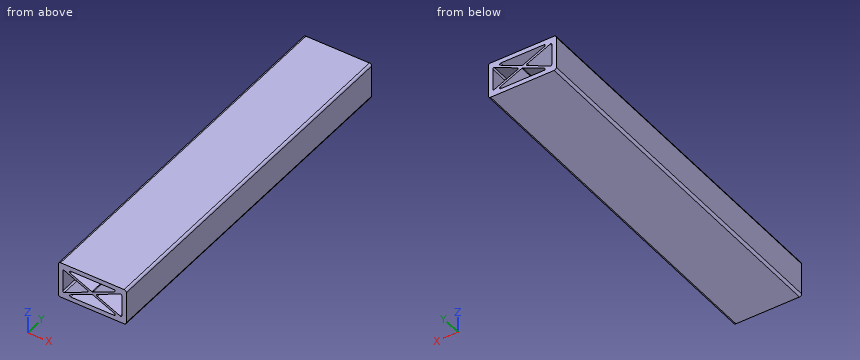
```python
from build123d import *

# Parameters (mm, degrees)
F0_W     = 150
F0_H     = 80
F1_DEPTH = 800
F3_DEPTH = 800.001
F4_R     = 2.5
F5_R     = 5


with BuildPart() as f1:
    # F0 (on Front) → F1 (new body)
    with BuildSketch(Plane.XZ):
        Rectangle(F0_W, F0_H)
    extrude(amount=F1_DEPTH)

    # F2 (on face) → F3 (cut, through all)
    with BuildSketch(Plane.XZ.offset(800)):
        Polygon((59.034241, 30), (-59.034241, 30), (0, 2.753427), align=None)
        Polygon((0, -2.753427), (-59.034241, -30), (59.034241, -30), align=None)
        Polygon((-5.965759, 0), (-65, 27.246573), (-65, -27.246573), align=None)
        Polygon((65, -27.246573), (65, 27.246573), (5.965759, 0), align=None)
    extrude(amount=-F3_DEPTH, mode=Mode.SUBTRACT)

    # F4
    f4_edges = [f1.edges().sort_by_distance(p)[0] for p in [
        (-59.034241, -400, 30),
        (5.965759, -400, 0),
        (0, -400, -2.753427),
        (-5.965759, -400, 0),
        (0, -400, 2.753427),
        (65, -400, -27.246573),
        (65, -400, 27.246573),
        (59.034241, -400, 30),
        (-65, -400, 27.246573),
        (-65, -400, -27.246573),
        (-59.034241, -400, -30),
        (59.034241, -400, -30),
    ]]
    fillet(f4_edges, radius=F4_R)

    # F5
    f5_edges = [f1.edges().sort_by_distance(p)[0] for p in [
        (-75, -400, 40),
        (-75, -400, -40),
        (75, -400, 40),
        (75, -400, -40),
    ]]
    fillet(f5_edges, radius=F5_R)


solid = f1.part
```
Work out the finished part from the listing and answer in its coordinate system (mm). Coordinates: 2 decimals unless noted, no trailing zeros. Order: outer loops, then holes, each group sorted by start corner. A loop starts at its lowest first (then second) coordinate and runs counter-clockwise, first axis right, second up. Notation, with made-up numbers: M -23.75,-28 L -0.75,-28 A12 ccw -0.75,-16 Z; hole C 18,-16.75 d1. An arc over 180 degrees is marked long. Use CSV: the item, a comma, the result in double quotes.
1) Consider line 1 (X direction, y = -409.5, z = -8); line 2 (X direction, y = -626, z = -18); line 3 (Z direction, x = -7, y = -378). Determine where each line is inside the solid, lowest interval first. Write a range as [from, to].
Worked out:
line 1,"x = [-75, -65], [-23.3, -11.37], [11.37, 23.3], [65, 75]"
line 2,"x = [-75, -65], [-44.97, -33.03], [33.03, 44.97], [65, 75]"
line 3,"z = [-40, -30], [-5.98, 5.98], [30, 40]"
2) Section A-A on y = -530.5 is taken. Count the separate pieces of the cut face and the enclosed holes in it, plus the area to 3 significant figures.
Worked out:
separate pieces,"1"
enclosed holes,"4"
area,"5,650 mm^2"
3) Section B-B on z = -16 is taken. Write down the section's boundary in (x, y), plus the area to 3 significant figures.
Worked out:
outline,"M -75,-800 L -65,-800 L -65,0 L -75,0 Z; M -40.63,-800 L -28.7,-800 L -28.7,0 L -40.63,0 Z; M 28.7,-800 L 40.63,-800 L 40.63,0 L 28.7,0 Z; M 65,-800 L 75,-800 L 75,0 L 65,0 Z"
area,"35,100 mm^2"
4) A flat-ended cylindrical pin translates along its axis: pin 1 Ø2 at (x, z) = (17, 28.5) entering from -Y. Find the tip coordinate at first contact, or state that the pin passes through.
Worked out:
pin 1,"passes through"
